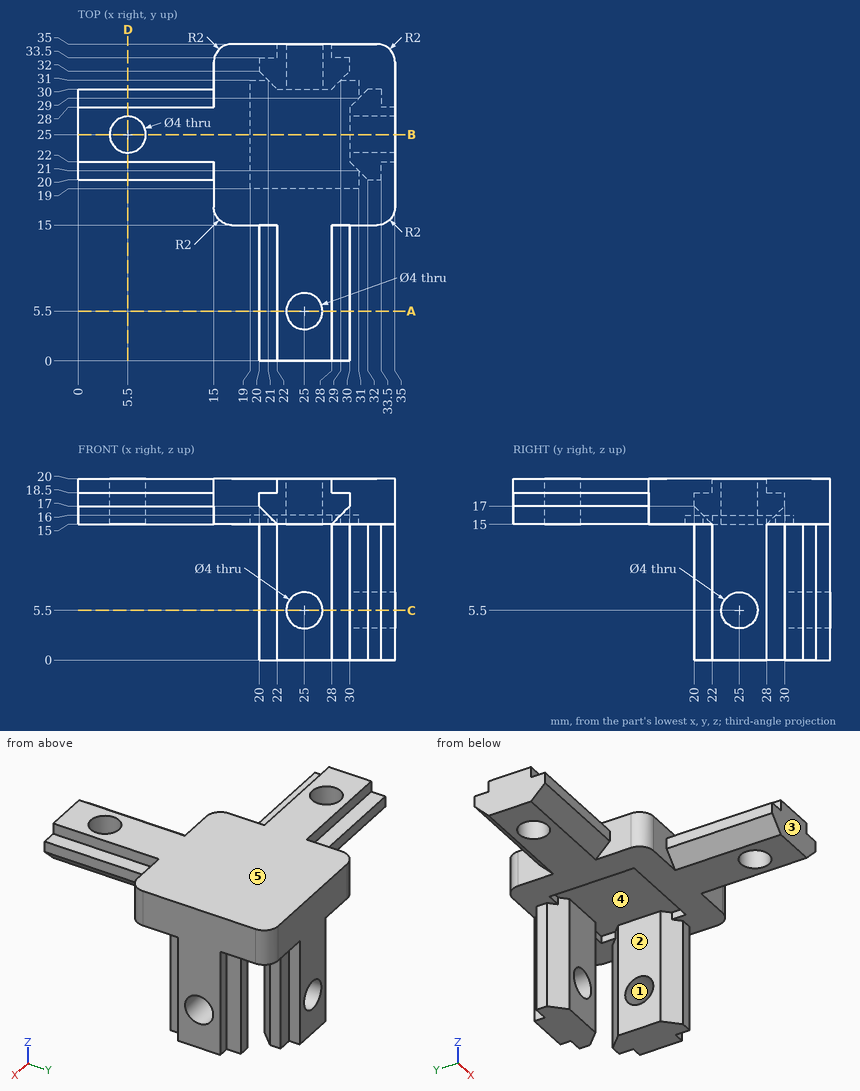
Drawing for the job (mm, zero at the part's lowest x, y, z). A direction names the side the tool comes from. Round coordinates to 2 decimals unless told otherwise and drop trailing zeros. Loops run counter-clockwise (first coordinate to the right, second up) from the corner with the lowest first, then second, coordinate; pieces in that order, holes last. Notation, with made-up numbers: M 33.5,78 L 75.5,78 A15 ccw 75.5,82 Z; hole C -3,71.25 d8. An arc over 180 degrees is marked long. Use a Markdown table: item, result. Add a question column.
(1) Cut at C-C (z = 5.5). Give the cut face in (x, y), and give its area (3 significant figures).
(2) Which spindle directions (+Z, -Z, +X, -X, +Y, -Y) get a long thin tool onto all of the face, cutting with end or side? Do the marked faces 1 and 2. Say none if no direction does.
(3) Cut at A-A (y = 5.5). Give the cut face in (x, z).
(4) Flat gauge pins, fed straight in: pin 1 (1.2 mm diameter, centred on y = 32.5, z = 8, fed in from -X); pin 2 (0.8 mm diameter, centred on x = 34, z = 7.5, fed in from +Y); pin 3 (1.5 mm diameter, centred on x = 10, z = 15, fed in from +Y). Where does each tip first touch, or does it go through?
(5) Cut at B-B (y = 25). Give the cut face in (x, z).
(6) Pull direction Y, two halves, no side cores. Call the marked faces 3, 4 and 5: +Y half, -Y half, draft (parallel to the pull), parting line (faces both ways), or undercut.
(7) Drill centre lines: line 1 (X direction, y = 32, z = 5.5); line 2 (Y direction, x = 25, z = 18.5); line 3 (Z direction, x = 25, y = 31). Where is each one in solid material? Low to high.
Geometry says:
| question | item | result |
|---|---|---|
| 1 | outline | M 20,32 L 22,30 L 23,30 L 23,35 L 22,35 L 22,33.5 L 20,33.5 Z; M 27,30 L 28,30 L 30,32 L 30,33.5 L 28,33.5 L 28,35 L 27,35 Z; M 30,22 L 32,20 L 33.5,20 L 33.5,22 L 35,22 L 35,23 L 30,23 Z; M 30,27 L 35,27 L 35,28 L 33.5,28 L 33.5,30 L 32,30 L 30,28 Z |
| 1 | area | 40.0 mm² |
| 2 | face 1 | +X, -X |
| 2 | face 2 | -Z |
| 3 | outline | M 20,17 L 22,15 L 23,15 L 23,20 L 22,20 L 22,18.5 L 20,18.5 Z; M 27,15 L 28,15 L 30,17 L 30,18.5 L 28,18.5 L 28,20 L 27,20 Z |
| 4 | pin 1 | stops at x = 20 |
| 4 | pin 2 | stops at y = 28 |
| 4 | pin 3 | stops at y = 28.75 |
| 5 | outline | M 0,15 L 3.5,15 L 3.5,20 L 0,20 Z; M 7.5,15 L 19,15 L 19,16 L 30,16 L 30,7.5 L 35,7.5 L 35,20 L 7.5,20 Z; M 30,0 L 35,0 L 35,3.5 L 30,3.5 Z |
| 6 | face 3 | -Y half |
| 6 | face 4 | undercut |
| 6 | face 5 | draft |
| 7 | line 1 | x = 20 to 23, 27 to 30 |
| 7 | line 2 | y = 0 to 3.5, 7.5 to 35 |
| 7 | line 3 | z = 0 to 3.5, 7.5 to 20 |
